Could you check a few things on this model? Use its own coordinates, in mm. Face numbers are marked on the shaded views. Coordinates: 2 decimals unless noted, no trailing zeros.
Item 1: For P1, Ø1.5, axis at x = -15.5, z = -15, coming from the -Y side; P2, Ø1.5, axis at y = 0, z = 5.5, coming from the +X side, each with a flat end and sliding along its axis, tell me the tip position at first contact or that it passes through.
Item 2: Thinking about a two-plate mould opening in X: for the marked faces 1 and 2, which applies, +X half, -X half, draft (parallel to the pull), parting line (faces both ways), or undercut?
Item 3: I want a section at B-B on x = 6. State how many separate pieces and enclosed holes the cut face has, then the cut area to 3 significant figures.
Item 4: If I drill on probe 1 along X at (y, z) = (1.65, 0); probe 2 along Z at (x, y) = (12.5, 1.3); probe 3 along X at (y, z) = (-0.45, 0), over which ranges is the centre line in solid material (lowest first)?
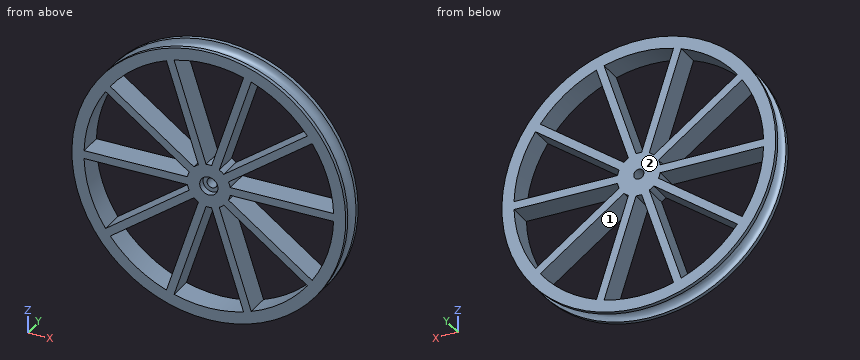
from build123d import *

# Parameters (mm, degrees)
INNERWHEEL_START                            = -0.79375
INNERWHEEL_OUTLINE_R                        = 4.28625
INNERWHEEL_OUTLINE_R_2                      = 3.01625
INNERWHEEL_DEPTH                            = 4.7625
CONNECTIONINNEROUTER_REACH                  = 43.498
CONNECTIONINNEROUTER_END_RADIUS             = 24.60625
SKETCH3_W                                   = 1.5875
SKETCH3_H                                   = 4.7625
CONNECTIONINNEROUTER_DIRECTION_2_REACH      = 43.498
CONNECTIONINNEROUTER_DIRECTION_2_END_RADIUS = 4.28625
CIRCULARPATTERN_COUNT                       = 10
SKETCH4_R                                   = 3.01625
FILLHOLE_DEPTH                              = 4.7625
M2SCREWHOLE_REACH                           = 40.462
M2SCREWDHOLE_R                              = 1
M2SCREWDKHEAD_R                             = 1.8
M2SCREWHEAD_DEPTH                           = 1.28
FILLET_2_R                                  = 1.5875


# Read off the part's stored shape, not the designer's step: InnerWheel
with BuildPart() as part:
    # OuterWheelSketch → OuterWheel (revolve)
    with BuildSketch(Plane.XY, mode=Mode.PRIVATE) as outerwheel_sk:
        Polygon((-25.4, 0), (-26.9875, 0), (-26.9875, -0.79375), (-24.60625, -0.79375), (-24.60625, 3.96875), (-26.9875, 3.96875), (-26.9875, 3.175), (-25.4, 3.175), align=None)
    revolve(outerwheel_sk.sketch.rotate(Axis((0, -1.962659061, 0), (0, 1, 0)), 270), axis=Axis((0, -1.962659061, 0), (0, 1, 0)))



with BuildPart() as body_2:
    # InnerWheel outline → InnerWheel (new body)
    with BuildSketch(Plane(origin=(0, 0, 0), x_dir=(1, 0, 0), z_dir=(0, 1, 0)).offset(INNERWHEEL_START)):
        Circle(INNERWHEEL_OUTLINE_R)
        Circle(INNERWHEEL_OUTLINE_R_2, mode=Mode.SUBTRACT)
    extrude(amount=INNERWHEEL_DEPTH)


with BuildPart() as part_1:
    add(part.part)

    add(body_2.part)  # ConnectionInnerOuter merges body 2
    # ConnectionInnerOuter: up to this cylinder (the profile starts inside it)
    connectioninnerouter_end = Plane(origin=(0, 1.5875, 0), z_dir=(0, -1, 0)) * Cylinder(CONNECTIONINNEROUTER_END_RADIUS, 137.2085, mode=Mode.PRIVATE)
    # Sketch3 → ConnectionInnerOuter (add, up to the surface)
    with BuildSketch(Plane(origin=(4.28625, 0, 0), x_dir=(0, 0, -1), z_dir=(1, 0, 0)), mode=Mode.PRIVATE) as connectioninnerouter_sk1:
        with Locations((0, 1.5875)):
            Rectangle(SKETCH3_W, SKETCH3_H)
    connectioninnerouter_tool1 = extrude(connectioninnerouter_sk1.sketch, amount=CONNECTIONINNEROUTER_REACH, mode=Mode.PRIVATE) & connectioninnerouter_end
    connectioninnerouter = connectioninnerouter_tool1.solids().sort_by_distance((4.28625, 1.5875, 0))[0]
    add(connectioninnerouter)

    # ConnectionInnerOuter direction 2: up to this cylinder (the profile starts outside it)
    connectioninnerouter_direction_2_end = Plane(origin=(0, 1.5875, 0), z_dir=(0, -1, 0)) * Cylinder(CONNECTIONINNEROUTER_DIRECTION_2_END_RADIUS, 96.5685, mode=Mode.PRIVATE)
    # Sketch3 → ConnectionInnerOuter direction 2 (add, up to the surface)
    with BuildSketch(Plane(origin=(4.28625, 0, 0), x_dir=(0, 0, -1), z_dir=(1, 0, 0)), mode=Mode.PRIVATE) as connectioninnerouter_direction_2_sk1:
        with Locations((0, 1.5875)):
            Rectangle(SKETCH3_W, SKETCH3_H)
    connectioninnerouter_direction_2_tool1 = extrude(connectioninnerouter_direction_2_sk1.sketch, amount=-CONNECTIONINNEROUTER_DIRECTION_2_REACH, mode=Mode.PRIVATE) - connectioninnerouter_direction_2_end
    connectioninnerouter_direction_2 = connectioninnerouter_direction_2_tool1.solids().sort_by_distance((4.28625, 1.5875, 0))[0] + connectioninnerouter_direction_2_tool1.solids().sort_by_distance((4.28625, 1.5875, 0))[1]
    add(connectioninnerouter_direction_2)
    connectioninnerouter = connectioninnerouter + connectioninnerouter_direction_2  # both directions under the feature's name, for the pattern or mirror that repeats it

    # CircularPattern: ConnectionInnerOuter ×10 about axis
    circularpattern_axis = Axis((0, 0, 0), (0, 1, 0))
    for i in range(1, CIRCULARPATTERN_COUNT):
        add(connectioninnerouter.rotate(circularpattern_axis, i * 360 / CIRCULARPATTERN_COUNT))

    # Sketch4 → FillHole (add)
    with BuildSketch(Plane(origin=(0, -0.79375, 0), x_dir=(-1, 0, 0), z_dir=(0, -1, 0))):
        Circle(SKETCH4_R)
    extrude(amount=-FILLHOLE_DEPTH)

    # M2ScrewDHole → M2ScrewHole (cut, up to next)
    with BuildSketch(Plane(origin=(0, -0.79375, 0), x_dir=(-1, 0, 0), z_dir=(0, -1, 0)), mode=Mode.PRIVATE) as m2screwhole_sk1:
        with Locations(Location((0, 0, 0), (0, 0, 90))):
            Circle(M2SCREWDHOLE_R)
    m2screwhole_tool1 = extrude(m2screwhole_sk1.sketch, amount=-M2SCREWHOLE_REACH, mode=Mode.PRIVATE) & part_1.part
    add(m2screwhole_tool1.solids().sort_by_distance((0, -0.79375, 0))[0], mode=Mode.SUBTRACT)

    # M2ScrewDKHead → M2ScrewHead (cut)
    with BuildSketch(Plane(origin=(0, -0.79375, 0), x_dir=(-1, 0, 0), z_dir=(0, -1, 0))):
        with Locations(Location((0, 0, 0), (0, 0, 90))):
            Circle(M2SCREWDKHEAD_R)
    extrude(amount=-M2SCREWHEAD_DEPTH, mode=Mode.SUBTRACT)

    # Fillet 2
    fillet_2_edges = [part_1.edges().sort_by_distance(p)[0] for p in [
        (0, 0, 25.4),
        (0, 3.175, 25.4),
    ]]
    fillet(fillet_2_edges, radius=FILLET_2_R - 0.0001)  # a hair under: the kernel refuses the full size


solid = part_1.part
Response values:
1. P1: passes through
1. P2: stops at x = 26.57
2. face 1: undercut
2. face 2: draft
3. separate pieces: 7
3. enclosed holes: 0
3. area: 90.4 mm2
4. probe 1: x = -25.4 to -1, 1 to 25.4
4. probe 2: z = -22.14 to -21.19, -10.06 to -8.1, -0.79 to 0.79, 8.1 to 10.06, 21.19 to 22.14
4. probe 3: x = -26.99 to -1.8, 1.8 to 26.99
